Study the drawing (mm; zero at the part's minimum x, y, z) and answer. Coordinates: 2 decimals unless noted, no trailing zeros. Loops run counter-clockwise (first coordinate to the right, second up) from the corner with the lowest first, then second, coordinate; pieces in that order, holes last. Notation, with made-up numbers: M -9.75,85 L 43.25,85 A14 ccw 43.25,89 Z; hole C 78,46 d7. An arc over 180 degrees is marked long. Use one line per item in the form item = value. Start each with the question number.
1. Find the intervals of material crossed by probe 1 along Y at (x, z) = (4.5, 7.25); probe 2 along X at (y, z) = (3.5, 5); probe 3 along Y at (x, z) = (2.5, 7.5), in increasing order. Write a range as [from, to].
2. Flat-ended cylindrical pins translate along their axes: pin 1 (1.5 mm diameter, centred on x = 2, z = 3, fed in from +Y); pin 2 (1.5 mm diameter, centred on x = 6.5, z = 5, fed in from +Y); pin 3 (4.5 mm diameter, centred on x = 4.5, y = 4.5, fed in from +Z). Find the tip coordinate at first contact, or state that the pin passes through.
3. The part is cut by section A-A (y = 4.5). Give the vertices of the cut face in (x, z), plus the area to 3 significant figures.
4. The part is cut by section C-C (z = 2.75). Give the vertices of the cut face in (x, y), plus the area to 3 significant figures.
5. For a pull along X with two mould halves and no side action, classify the marked faces 1, 2 and 3 as released by +X, released by -X, zero draft, split by the parting line, or undercut.
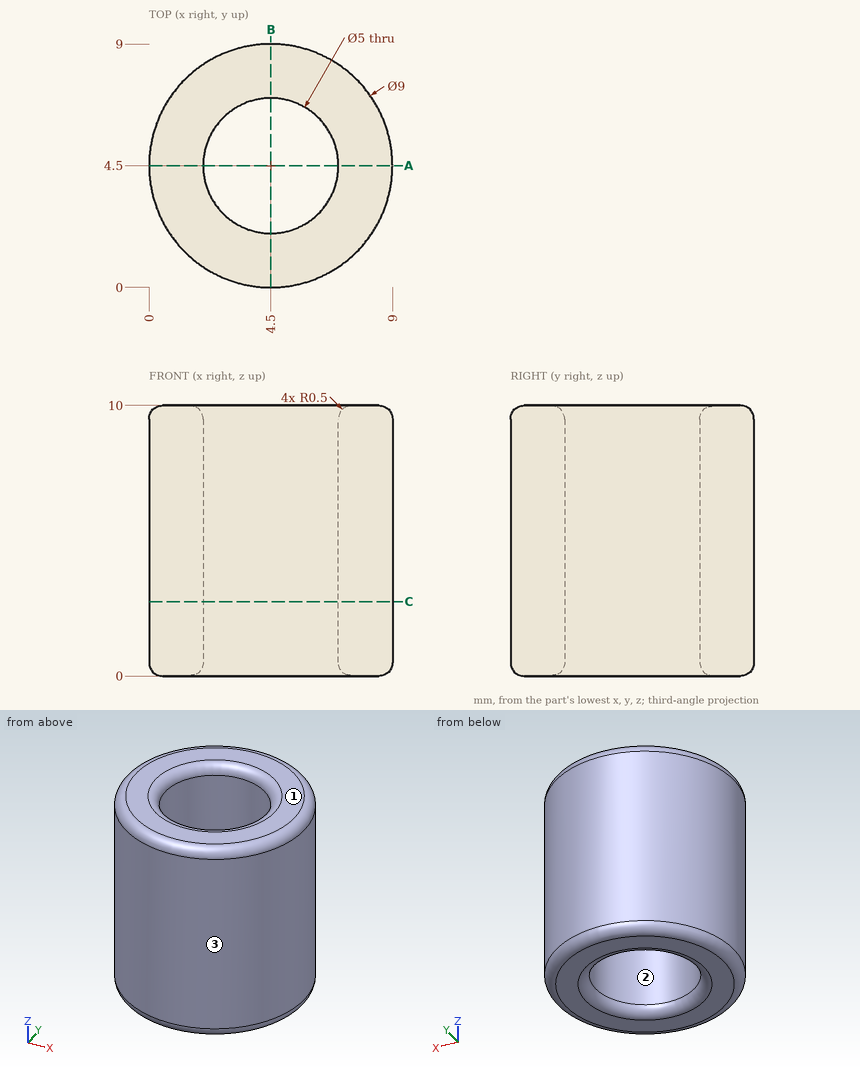
Computed values:
q1.probe_1 = [0, 2], [7, 9]
q1.probe_2 = [0.11, 2.21], [6.79, 8.89]
q1.probe_3 = [0.47, 3], [6, 8.53]
q2.pin_1 = 8.65
q2.pin_2 = 8.82
q2.pin_3 = through
q3.outline = M 0,0.5 A0.5 ccw 0.5,0 L 1.5,0 A0.5 ccw 2,0.5 L 2,9.5 A0.5 ccw 1.5,10 L 0.5,10 A0.5 ccw 0,9.5 Z; M 7,0.5 A0.5 ccw 7.5,0 L 8.5,0 A0.5 ccw 9,0.5 L 9,9.5 A0.5 ccw 8.5,10 L 7.5,10 A0.5 ccw 7,9.5 Z
q3.area = 39.6 mm²
q4.outline = C 4.5,4.5 d9; hole C 4.5,4.5 d5
q4.area = 44.0 mm²
q5.face_1 = zero draft
q5.face_2 = undercut
q5.face_3 = split by the parting line
